The model under review builds one solid part; all positions refer to its coordinate system, in mm. A direction names the side the tool comes from. Round coordinates to 2 decimals unless told otherwise and drop trailing zeros. Loops run counter-clockwise (first coordinate to the right, second up) from the corner with the lowest first, then second, coordinate; pieces in that order, holes last. Notation, with made-up numbers: (50.5, -26) -> (54.5, -26) arc R5 ccw to (54.5, -22) -> close; hole circle Ø7 at (16, 21.25). An arc over 180 degrees is marked (long way). Use a Markdown table: item, result. Add a question column.
1) Wall thickness on probe 1 along Y at (x, z) = (-50, -3.5); probe 2 along Y at (x, z) = (-12, 6.25); probe 3 along Y at (x, z) = (59, -3.25): over which ranges is each line inside the solid? List them lowest first.
2) Mouldability with a two-part tool opening along Y and no side actions: class faces 4 (the cylindrical face through (-5.21, 39.66, 0.14)), 5 (the flat face through (-21.363, 15.798, 0.14)), 6 (the flat face through (50, 6, 5)) as released by +Y, released by -Y, zero draft, split by the parting line, or undercut.
3) For faces 1 (the flat face through (-48, 1, -5)), 2 (the flat face through (-24.228, 10.524, 0.14)), 3 (the flat face through (79.857, -33.551, 0.07)), list the 3-axis set-ups (+Z, -Z, +X, -X, +Y, -Y) from which the entire face can be reached by the end or side of a thin tool; tool diameter is ignored.
4) Consider section B-B on y = -65.5. Give the boundary of the cut face in (x, z).
5) Consider section C-C on x = 74.5. Give the boundary of the cut face in (y, z), plus the area to 3 significant figures.
6) Insertion check: pin 1 (10 mm diameter, centred on x = -27.5, z = 3, fed in from -Y); pin 2 (1.5 mm diameter, centred on x = -16, z = -5.5, fed in from +Y); pin 3 (12 mm diameter, centred on y = 26.5, z = -4, fed in from +X); pin 4 (6 mm diameter, centred on x = 17, y = -37, fed in from -Z). Each pin has a flat end and moves straight along its axis. Give the tip position at first contact, or say it passes through.
7) Consider section A-A on z = 8. State how many separate pieces and enclosed holes the cut face has, plus the area to 3 significant figures.
from build123d import *

# Parameters (mm, degrees)
SKETCH1_R             = 15
BOSS_EXTRUDE1_DEPTH   = 10
SKETCH1_R_2           = 20
BOSS_EXTRUDE1_2_DEPTH = 10
SKETCH1_R_3           = 40
SKETCH1_R_4           = 16
BOSS_EXTRUDE1_3_DEPTH = 10
SKETCH1_4_R           = 15
BOSS_EXTRUDE2_DEPTH   = 5


with BuildPart() as part:
    # Sketch1 → Boss-Extrude1 (new, symmetric)
    with BuildSketch(Plane.XY):
        with BuildLine():
            ThreePointArc((-88.964969944, 6.350583834), (-90, 0), (-88.964969944, -6.350583834))
            ThreePointArc((-88.964969944, -6.350583834), (-66.782811699, -19.739546586), (-50, 0))
            ThreePointArc((-50, 0), (-66.782811699, 19.739546586), (-88.964969944, 6.350583834))
        make_face()
        with Locations((-70, 0)):
            Circle(SKETCH1_R, mode=Mode.SUBTRACT)
    extrude(amount=BOSS_EXTRUDE1_DEPTH, both=True)



with BuildPart() as body_2:
    # Sketch1 → Boss-Extrude1 2 (new, symmetric)
    with BuildSketch(Plane.XY):
        with Locations((70, 0)):
            Circle(SKETCH1_R_2)
        with Locations((70, 0)):
            Circle(SKETCH1_R, mode=Mode.SUBTRACT)
    extrude(amount=BOSS_EXTRUDE1_2_DEPTH, both=True)


with BuildPart() as body_3:
    # Sketch1 → Boss-Extrude1 3 (new, symmetric)
    with BuildSketch(Plane.XY):
        Circle(SKETCH1_R_3)
        Circle(SKETCH1_R_4, mode=Mode.SUBTRACT)
        with BuildLine():
            Line((16.5, 12.990381057), (26.090759323, 18.527608533))
            ThreePointArc((26.090759323, 18.527608533), (16, 27.712812921), (3, 31.859064644))
            Line((3, 31.859064644), (3, 20.784609691))
            ThreePointArc((3, 20.784609691), (10.5, 18.186533479), (16.5, 12.990381057))
        make_face(mode=Mode.SUBTRACT)
        with BuildLine():
            Line((19.5, -7.794228634), (29.090759323, -13.331456111))
            ThreePointArc((29.090759323, -13.331456111), (32, 0), (29.090759323, 13.331456111))
            Line((29.090759323, 13.331456111), (19.5, 7.794228634))
            ThreePointArc((19.5, 7.794228634), (21, 0), (19.5, -7.794228634))
        make_face(mode=Mode.SUBTRACT)
        with BuildLine():
            Line((3, -20.784609691), (3, -31.859064644))
            ThreePointArc((3, -31.859064644), (16, -27.712812921), (26.090759323, -18.527608533))
            Line((26.090759323, -18.527608533), (16.5, -12.990381057))
            ThreePointArc((16.5, -12.990381057), (10.5, -18.186533479), (3, -20.784609691))
        make_face(mode=Mode.SUBTRACT)
        with BuildLine():
            Line((-3, 20.784609691), (-3, 31.859064644))
            ThreePointArc((-3, 31.859064644), (-16, 27.712812921), (-26.090759323, 18.527608533))
            Line((-26.090759323, 18.527608533), (-16.5, 12.990381057))
            ThreePointArc((-16.5, 12.990381057), (-10.5, 18.186533479), (-3, 20.784609691))
        make_face(mode=Mode.SUBTRACT)
        with BuildLine():
            ThreePointArc((-29.090759323, 13.331456111), (-32, 0), (-29.090759323, -13.331456111))
            Line((-29.090759323, -13.331456111), (-19.5, -7.794228634))
            ThreePointArc((-19.5, -7.794228634), (-21, 0), (-19.5, 7.794228634))
            Line((-19.5, 7.794228634), (-29.090759323, 13.331456111))
        make_face(mode=Mode.SUBTRACT)
        with BuildLine():
            ThreePointArc((-26.090759323, -18.527608533), (-16, -27.712812921), (-3, -31.859064644))
            Line((-3, -31.859064644), (-3, -20.784609691))
            ThreePointArc((-3, -20.784609691), (-10.5, -18.186533479), (-16.5, -12.990381057))
            Line((-16.5, -12.990381057), (-26.090759323, -18.527608533))
        make_face(mode=Mode.SUBTRACT)
    extrude(amount=BOSS_EXTRUDE1_3_DEPTH, both=True)


with BuildPart() as part_1:
    add(part.part)

    add(body_2.part)  # Boss-Extrude2 merges body 2

    add(body_3.part)  # Boss-Extrude2 merges body 3
    # Sketch1_4 → Boss-Extrude2 (add, symmetric)
    # profile 1 of 2: a face of its own
    with BuildSketch(Plane.XY):
        with BuildLine():
            Line((-88.964969944, -6.350583834), (-71, -60))
            ThreePointArc((-71, -60), (-50, -81), (-29, -60))
            ThreePointArc((-29, -60), (-22.304723723, -44.376428641), (-6.007722482, -39.546267467))
            ThreePointArc((-6.007722482, -39.546267467), (-40, 0), (-6.007722482, 39.546267467))
            ThreePointArc((-6.007722482, 39.546267467), (-22.304723723, 44.376428641), (-29, 60))
            ThreePointArc((-29, 60), (-50, 81), (-71, 60))
            Line((-71, 60), (-88.964969944, 6.350583834))
            ThreePointArc((-88.964969944, 6.350583834), (-66.782811699, 19.739546586), (-50, 0))
            ThreePointArc((-50, 0), (-66.782811699, -19.739546586), (-88.964969944, -6.350583834))
        make_face()
        with Locations((-50, -60)):
            Circle(SKETCH1_4_R, mode=Mode.SUBTRACT)
        with Locations((-50, 60)):
            Circle(SKETCH1_4_R, mode=Mode.SUBTRACT)
    # profile 2 of 2: a face of its own
    with BuildSketch(Plane.XY):
        with BuildLine():
            ThreePointArc((40, 0), (30.334047696, -26.073848016), (6.007722482, -39.546267467))
            ThreePointArc((6.007722482, -39.546267467), (22.304723723, -44.376428641), (29, -60))
            ThreePointArc((29, -60), (50, -81), (71, -60))
            Line((71, -60), (88.964969944, -6.350583834))
            ThreePointArc((88.964969944, -6.350583834), (50, 0), (88.964969944, 6.350583834))
            Line((88.964969944, 6.350583834), (71, 60))
            ThreePointArc((71, 60), (50, 81), (29, 60))
            ThreePointArc((29, 60), (22.304723723, 44.376428641), (6.007722482, 39.546267467))
            ThreePointArc((6.007722482, 39.546267467), (30.334047696, 26.073848016), (40, 0))
        make_face()
        with Locations((50, -60)):
            Circle(SKETCH1_4_R, mode=Mode.SUBTRACT)
        with Locations((50, 60)):
            Circle(SKETCH1_4_R, mode=Mode.SUBTRACT)
    extrude(amount=BOSS_EXTRUDE2_DEPTH, both=True)


solid = part_1.part
Result set:
| question | item | result |
|---|---|---|
| 1 | probe 1 | -81 to -75, -45 to 45, 75 to 81 |
| 1 | probe 2 | -38.16 to -29.66, -17.23 to -10.58, 10.58 to 17.23, 29.66 to 38.16 |
| 1 | probe 3 | -78.97 to -72, -48 to -10.2, 10.2 to 48, 72 to 78.97 |
| 2 | face 4 | split by the parting line |
| 2 | face 5 | undercut |
| 2 | face 6 | zero draft |
| 3 | face 1 | -Z |
| 3 | face 2 | +Z, -Z |
| 3 | face 3 | +Z, -Z, +X, -Y |
| 4 | outline | (-70.27, -5) -> (-63.96, -5) -> (-63.96, 5) -> (-70.27, 5) -> close; (-36.04, -5) -> (-29.73, -5) -> (-29.73, 5) -> (-36.04, 5) -> close; (29.73, -5) -> (36.04, -5) -> (36.04, 5) -> (29.73, 5) -> close; (63.96, -5) -> (70.27, -5) -> (70.27, 5) -> (63.96, 5) -> close |
| 5 | outline | (-49.55, -5) -> (-19.49, -5) -> (-19.49, -10) -> (-14.31, -10) -> (-14.31, 10) -> (-19.49, 10) -> (-19.49, 5) -> (-49.55, 5) -> close; (14.31, -10) -> (19.49, -10) -> (19.49, -5) -> (49.55, -5) -> (49.55, 5) -> (19.49, 5) -> (19.49, 10) -> (14.31, 10) -> close |
| 5 | area | 808 mm2 |
| 6 | pin 1 | y = -71.61 |
| 6 | pin 2 | y = 40.8 |
| 6 | pin 3 | x = 84.23 |
| 6 | pin 4 | z = -10 |
| 7 | separate pieces | 3 |
| 7 | enclosed holes | 9 |
| 7 | area | 3,890 mm2 |
